from build123d import *

# Parameters (mm, degrees)
SKETCH2_R           = 6.5000000000000036
BOSS_EXTRUDE2_DEPTH = 40
CIRPATTERN15_COUNT  = 6
CHAMFER1_SIZE       = 1.5
FILLET1_R           = 25
FILLET2_R           = 15


with BuildPart() as part:
    # Sketch1 → Revolve1 (revolve)
    with BuildSketch(Plane.XY):
        Polygon((2.8e-16, 75), (0, 0), (-30, 0), (-30, 29.999999999999996), (-50.00000000000002, 29.999999999999993), (-50.00000000000002, 34.99999999999999), (-90.00000000000003, 34.99999999999999), (-90.00000000000003, 54.99999999999999), (-40.000000000000014, 54.99999999999999), (-40, 105), (-30.000000000000004, 105), (-30, 75), align=None)
    revolve(axis=Axis((2.8e-16, 75, 0), (0, -1, 0)))

    # Sketch2 → Boss-Extrude2 (add)
    with BuildSketch(Plane(origin=(2.1e-16, 54.99999999999999, 0), x_dir=(1, 0, 0), z_dir=(0, 1, 0))):
        with Locations(Location((0, 81, 0), (0, 0, 180))):
            Circle(SKETCH2_R)
    boss_extrude2 = extrude(amount=-BOSS_EXTRUDE2_DEPTH)

    # CirPattern15: Boss-Extrude2 ×6 about axis
    cirpattern15_axis = Axis((9.552e-14, 0, 1.87e-15), (0, 1, 0))
    for i in range(1, CIRPATTERN15_COUNT):
        add(boss_extrude2.rotate(cirpattern15_axis, i * 360 / CIRPATTERN15_COUNT))

    # Chamfer1
    chamfer1_edges = [part.edges().sort_by_distance(p)[0] for p in [
        (6.5000000000000036, 14.999999999999993, -81),
        (73.39805770653957, 14.999999999999993, -34.870834875401236),
        (66.89805770653965, 14.999999999999993, 46.129165124598806),
        (-6.499999999999822, 14.999999999999993, 81),
        (-73.39805770653939, 14.999999999999993, 34.87083487540121),
        (-66.89805770653949, 14.999999999999993, -46.12916512459878),
    ]]
    chamfer(chamfer1_edges, length=CHAMFER1_SIZE)

    # Fillet1
    # the kernel refuses this fillet: 25 mm, written as the material it adds along each edge
    with BuildSketch(Plane(origin=(1.1e-16, 30, 0), x_dir=(-1, 0, 0), z_dir=(0, 0, 1))) as fillet1_piece_1:
        with BuildLine():
            CenterArc((55, 24.494897427831788), FILLET1_R, 180, 78.46304096718455)
            Line((30, 24.494897427831788), (29.5, 24.494897427831788))
            Line((29.5, 24.494897427831788), (29.5, 0))
            Line((29.5, 0), (30, -0.5))
            ThreePointArc((30, -0.5), (40.000000000000014, -0.5), (49.90000000000002, -0.4898979485566315))
            Line((49.90000000000002, -0.4898979485566315), (50.00000000000002, 3.55e-15))
        make_face()
    revolve(axis=Axis((1.1e-16, 30, 0), (0, -1, 0)))
    with BuildSketch(Plane(origin=(2.1e-16, 54.99999999999999, 0), x_dir=(-1, 0, 0), z_dir=(0, 0, 1))) as fillet1_piece_2:
        with BuildLine():
            CenterArc((40.000000000000014 + FILLET1_R, -FILLET1_R), FILLET1_R, 90, 89.99999999999997)
            Line((40.000000000000014, -FILLET1_R), (40.000000000000014 - FILLET1_R * 0.02, -FILLET1_R))
            Line((40.000000000000014 - FILLET1_R * 0.02, -FILLET1_R), (40.000000000000014 - FILLET1_R * 0.02, FILLET1_R * 0.02))
            Line((40.000000000000014 - FILLET1_R * 0.02, FILLET1_R * 0.02), (40.000000000000014 + FILLET1_R, FILLET1_R * 0.02))
            Line((40.000000000000014 + FILLET1_R, FILLET1_R * 0.02), (40.000000000000014 + FILLET1_R, -7.11e-15))
        make_face()
    revolve(axis=Axis((2.1e-16, 54.99999999999999, 0), (0, -1, 0)))

    # Fillet2
    fillet2_edges = [part.edges().sort_by_distance(p)[0] for p in [
        (30, -1.1e-16, -1.7e-14),
    ]]
    fillet(fillet2_edges, radius=FILLET2_R)


solid = part.part
Design review of the part built by this model. Coordinates are the model's own, in mm. A direction names the side the tool comes from. Round coordinates to 2 decimals unless told otherwise and drop trailing zeros. Write each loop counter-clockwise with the first axis right and the second up, starting at its lowest first coordinate (ties: lowest second). Pieces come first, ordered by that corner, then holes.
Item 1: Consider section C-C on y = 62. Give the boundary of the cut face in (x, z), and give its area (3 significant figures).
Item 2: For faces 4 (the cylindrical face through (29.97, 89.79, -1.32)), 5 (the cylindrical face through (-63.654, 25.879, 40.786)), 6 (the flat face through (0, 15, 81)), 7 (the flat face through (70, 15, -40)), list the 3-axis set-ups (+Z, -Z, +X, -X, +Y, -Y) from which the entire face can be reached by the end or side of a thin tool; tool diameter is ignored.
Item 3: Consider section A-A on y = 39. Give the boundary of the cut face in (x, z), and give its area (3 significant figures).
Item 4: Wall thickness on L1, parallel to Z at x = 0, y = 87.75; L2, parallel to Y at x = 14, z = 5.5: over which ranges is each line inside the solid? List them lowest first.
Item 5: Consider section B-B on z = -81. Give the boundary of the cut face in (x, y), and give its area (3 significant figures).
Item 6: For pin 1 Ø10 at (x, y) = (29, 22.5) entering from +Z; pin 2 Ø12 at (x, y) = (-24.5, 58.5) entering from -Z; pin 3 Ø11 at (x, z) = (69, 41) entering from -Y, all flat-tipped, find the tip position at first contact; note any pin that passes through.
Item 7: Draft analysis for pull direction Z (two halves, no side actions). For faces 1 (the cylindrical face through (-1.409, 25.879, 87.345)), 2 (the flat face through (-70, 15, -41)), 3 (the cylindrical face through (-18.458, 92.675, 35.487)), state which applies: released by +Z, released by -Z, zero draft, split by the parting line, or undercut.
Check values:
1. outline: circle Ø95.3 at (0, 0)
1. area: 7,130 mm2
2. face 4: +Y
2. face 5: -Y
2. face 6: +Z, +X, -X, -Y
2. face 7: +Z, -Z, +X, -X, -Y
3. outline: circle Ø180 at (0, 0)
3. area: 25,400 mm2
4. L1: z = -40 to -30, 30 to 40
4. L2: y = 0 to 75
5. outline: (-39.23, 35) - (-6.5, 35) - (-6.5, 16.5) - (-5, 15) - (5, 15) - (6.5, 16.5) - (6.5, 35) - (39.23, 35) - (39.23, 55) - (-39.23, 55) - close
5. area: 1,830 mm2
6. pin 1: stops at z = 32.68
6. pin 2: stops at z = -87.83
6. pin 3: stops at y = 15
7. face 1: undercut
7. face 2: zero draft
7. face 3: split by the parting line
